from build123d import *

# Parameters (mm, degrees)
CROQUIS1_R              = 44
SALIENTE_EXTRUIR1_DEPTH = 20
CROQUIS3_R              = 2.1
CORTAR_EXTRUIR3_DEPTH   = 81.199750623
CORTAR_EXTRUIR5_DEPTH   = 3.5
VACIADO1_START          = 3
VACIADO1_DEPTH          = 17
VACIADO1_START_2        = 6.5
VACIADO1_2_DEPTH        = 13.5
CROQUIS2_R              = 3
CORTAR_EXTRUIR1_DEPTH   = 66.360538553
CROQUIS4_R              = 42.5
CORTAR_EXTRUIR4_DEPTH   = 2
CHAFL_N1_SIZE           = 2


# Read off the part's stored shape, not the designer's step: Vaciado1
with BuildPart() as part:
    # Croquis1 → Saliente-Extruir1 (new body)
    with BuildSketch(Plane(origin=(0, 0, 0), x_dir=(1, 0, 0), z_dir=(0, 1, 0))):
        with Locations(Location((0, 0, 0), (0, 0, 270))):
            Circle(CROQUIS1_R)
    extrude(amount=SALIENTE_EXTRUIR1_DEPTH)

    # Croquis3 → Cortar-Extruir3 (cut, through all)
    with BuildSketch(Plane(origin=(0, 20, -20), x_dir=(1, 0, 0), z_dir=(0, -1, 0))):
        with Locations(Location((-40, 20, 0), (0, 0, 270))):
            Circle(CROQUIS3_R)
        with Locations(Location((0, 60, 0), (0, 0, 270))):
            Circle(CROQUIS3_R)
        with Locations(Location((40, 20, 0), (0, 0, 270))):
            Circle(CROQUIS3_R)
        with Locations(Location((0, -20, 0), (0, 0, 270))):
            Circle(CROQUIS3_R)
    extrude(amount=CORTAR_EXTRUIR3_DEPTH, mode=Mode.SUBTRACT)

    # Croquis5 → Cortar-Extruir5 (cut)
    with BuildSketch(Plane.XZ):
        Polygon((40, -3.92598183), (43.4, -1.962990915), (43.4, 1.962990915), (40, 3.92598183), (36.6, 1.962990915), (36.6, -1.962990915), align=None)
        Polygon((3.92598183, 40), (1.962990915, 43.4), (-1.962990915, 43.4), (-3.92598183, 40), (-1.962990915, 36.6), (1.962990915, 36.6), align=None)
        Polygon((-3.92598183, -40), (-1.962990915, -43.4), (1.962990915, -43.4), (3.92598183, -40), (1.962990915, -36.6), (-1.962990915, -36.6), align=None)
        Polygon((-40, 3.92598183), (-43.4, 1.962990915), (-43.4, -1.962990915), (-40, -3.92598183), (-36.6, -1.962990915), (-36.6, 1.962990915), align=None)
    extrude(amount=-CORTAR_EXTRUIR5_DEPTH, mode=Mode.SUBTRACT)

    # Vaciado1 outline → Vaciado1 (cut)
    with BuildSketch(Plane(origin=(0, 0, 0), x_dir=(1, 0, 0), z_dir=(0, 1, 0)).offset(VACIADO1_START)):
        with BuildLine():
            ThreePointArc((-7.178364733, 40.366707567), (-28.991378029, 28.991378029), (-40.366707567, 7.178364733))
            Line((-40.366707567, 7.178364733), (-40, 7.390083446))
            Line((-40, 7.390083446), (-33.6, 3.695041723))
            Line((-33.6, 3.695041723), (-33.6, -3.695041723))
            Line((-33.6, -3.695041723), (-40, -7.390083446))
            Line((-40, -7.390083446), (-40.366707567, -7.178364733))
            ThreePointArc((-40.366707567, -7.178364733), (-28.991378029, -28.991378029), (-7.178364733, -40.366707567))
            Line((-7.178364733, -40.366707567), (-7.390083446, -40))
            Line((-7.390083446, -40), (-3.695041723, -33.6))
            Line((-3.695041723, -33.6), (3.695041723, -33.6))
            Line((3.695041723, -33.6), (7.390083446, -40))
            Line((7.390083446, -40), (7.178364733, -40.366707567))
            ThreePointArc((7.178364733, -40.366707567), (28.991378029, -28.991378029), (40.366707567, -7.178364733))
            Line((40.366707567, -7.178364733), (40, -7.390083446))
            Line((40, -7.390083446), (33.6, -3.695041723))
            Line((33.6, -3.695041723), (33.6, 3.695041723))
            Line((33.6, 3.695041723), (40, 7.390083446))
            Line((40, 7.390083446), (40.366707567, 7.178364733))
            ThreePointArc((40.366707567, 7.178364733), (28.991378029, 28.991378029), (7.178364733, 40.366707567))
            Line((7.178364733, 40.366707567), (7.390083446, 40))
            Line((7.390083446, 40), (3.695041723, 33.6))
            Line((3.695041723, 33.6), (-3.695041723, 33.6))
            Line((-3.695041723, 33.6), (-7.390083446, 40))
            Line((-7.390083446, 40), (-7.178364733, 40.366707567))
        make_face()
    extrude(amount=VACIADO1_DEPTH, mode=Mode.SUBTRACT)

    # Vaciado1 2 outline → Vaciado1 2 (cut)
    with BuildSketch(Plane(origin=(0, 0, 0), x_dir=(1, 0, 0), z_dir=(0, 1, 0)).offset(VACIADO1_START_2)):
        with BuildLine():
            ThreePointArc((-40.366707567, 7.178364733), (-40.540965383, 6.118016497), (-40.687375, 5.053465703))
            ThreePointArc((-40.687375, 5.053465703), (-34.9, 0), (-40.687375, -5.053465703))
            ThreePointArc((-40.687375, -5.053465703), (-40.540965383, -6.118016497), (-40.366707567, -7.178364733))
            Line((-40.366707567, -7.178364733), (-40, -7.390083446))
            Line((-40, -7.390083446), (-33.6, -3.695041723))
            Line((-33.6, -3.695041723), (-33.6, 3.695041723))
            Line((-33.6, 3.695041723), (-40, 7.390083446))
            Line((-40, 7.390083446), (-40.366707567, 7.178364733))
        make_face()
        with BuildLine():
            ThreePointArc((-5.053465703, 40.687375), (-6.118016497, 40.540965383), (-7.178364733, 40.366707567))
            Line((-7.178364733, 40.366707567), (-7.390083446, 40))
            Line((-7.390083446, 40), (-3.695041723, 33.6))
            Line((-3.695041723, 33.6), (3.695041723, 33.6))
            Line((3.695041723, 33.6), (7.390083446, 40))
            Line((7.390083446, 40), (7.178364733, 40.366707567))
            ThreePointArc((7.178364733, 40.366707567), (6.118016497, 40.540965383), (5.053465703, 40.687375))
            ThreePointArc((5.053465703, 40.687375), (0, 34.9), (-5.053465703, 40.687375))
        make_face()
        with BuildLine():
            Line((-7.390083446, -40), (-7.178364733, -40.366707567))
            ThreePointArc((-7.178364733, -40.366707567), (-6.118016497, -40.540965383), (-5.053465703, -40.687375))
            ThreePointArc((-5.053465703, -40.687375), (0, -34.9), (5.053465703, -40.687375))
            ThreePointArc((5.053465703, -40.687375), (6.118016497, -40.540965383), (7.178364733, -40.366707567))
            Line((7.178364733, -40.366707567), (7.390083446, -40))
            Line((7.390083446, -40), (3.695041723, -33.6))
            Line((3.695041723, -33.6), (-3.695041723, -33.6))
            Line((-3.695041723, -33.6), (-7.390083446, -40))
        make_face()
        with BuildLine():
            ThreePointArc((40.687375, 5.053465703), (40.540965383, 6.118016497), (40.366707567, 7.178364733))
            Line((40.366707567, 7.178364733), (40, 7.390083446))
            Line((40, 7.390083446), (33.6, 3.695041723))
            Line((33.6, 3.695041723), (33.6, -3.695041723))
            Line((33.6, -3.695041723), (40, -7.390083446))
            Line((40, -7.390083446), (40.366707567, -7.178364733))
            ThreePointArc((40.366707567, -7.178364733), (40.540965383, -6.118016497), (40.687375, -5.053465703))
            ThreePointArc((40.687375, -5.053465703), (34.9, 0), (40.687375, 5.053465703))
        make_face()
    extrude(amount=VACIADO1_2_DEPTH, mode=Mode.SUBTRACT)

    # Croquis2 → Cortar-Extruir1 (cut, through all)
    with BuildSketch(Plane.XZ):
        with Locations(Location((0, 25, 0), (0, 0, 270))):
            Circle(CROQUIS2_R)
        with Locations(Location((25, 0, 0), (0, 0, 270))):
            Circle(CROQUIS2_R)
        with Locations(Location((0, -25, 0), (0, 0, 270))):
            Circle(CROQUIS2_R)
        with Locations(Location((-25, 0, 0), (0, 0, 270))):
            Circle(CROQUIS2_R)
    extrude(amount=-CORTAR_EXTRUIR1_DEPTH, mode=Mode.SUBTRACT)

    # Croquis4 → Cortar-Extruir4 (cut)
    with BuildSketch(Plane(origin=(0, 20, 0), x_dir=(1, 0, 0), z_dir=(0, 1, 0))):
        with Locations(Location((0, 0, 0), (0, 0, 270))):
            Circle(CROQUIS4_R)
    extrude(amount=-CORTAR_EXTRUIR4_DEPTH, mode=Mode.SUBTRACT)

    # Chaflán1
    chafl_n1_edges = [part.edges().sort_by_distance(p)[0] for p in [
        (-28.991378029, 3, 28.991378029),
    ]]
    chamfer(chafl_n1_edges, length=CHAFL_N1_SIZE)


solid = part.part
Build history of the part. All positions in model axes, mm. A direction names the side the tool comes from. Round coordinates to 2 decimals unless told otherwise and drop trailing zeros. Loops run counter-clockwise (first coordinate to the right, second up) from the corner with the lowest first, then second, coordinate; pieces in that order, holes last. Notation, with made-up numbers: (37, -38.5) -> (54, -38.5) arc R22 ccw to (54, -20.5) -> close; hole circle Ø2 at (18.25, 53.25). An arc over 180 degrees is marked (long way). Answer in a Markdown table with one row per item.
Item 1: Saw through at C-C (z = -25). Write the cut outline in (x, y), and give its area (3 significant figures).
Answers below:
| item | result |
|---|---|
| outline | (-36.21, 0) -> (-3, 0) -> (-3, 3) -> (-32.5, 3) -> (-32.5, 18) -> (-34.37, 18) -> (-34.37, 20) -> (-36.21, 20) -> close; (3, 0) -> (36.21, 0) -> (36.21, 20) -> (34.37, 20) -> (34.37, 18) -> (32.5, 18) -> (32.5, 3) -> (3, 3) -> close |
| area | 318 mm² |
Item 2: Mould opens along Z. For faces 1 (the flat face through (23, 20, -36)), 2 (the flat face through (-5.568, 4.726, 36.845)) say: +Z half, -Z half, draft (parallel to the pull), parting line (faces both ways), or undercut.
Answers below:
| item | result |
|---|---|
| face 1 | draft |
| face 2 | undercut |
Item 3: Pin check, flat tips, straight feed: pin 1 (12 mm diameter, centred on x = 12.5, z = 3.5, fed in from +Y); pin 2 (4 mm diameter, centred on x = -34.5, y = 4, fed in from +Z); pin 3 (3 mm diameter, centred on y = 7, z = -26.5, fed in from -X). Stop position of each tip, or through.
Answers below:
| item | result |
|---|---|
| pin 1 | stops at y = 3 |
| pin 2 | stops at z = 29.66 |
| pin 3 | stops at x = -36.21 |
Item 4: Which spindle directions (+Z, -Z, +X, -X, +Y, -Y) get a long thin tool onto all of the face, cutting with end or side? Do faces 3 (the flat face through (36.845, 4.726, 5.568)), 4 (the cylindrical face through (25.9, 1.48, -2.86)), 5 (the flat face through (2.958, 1.726, -38.324)). Say none if no direction does.
Answers below:
| item | result |
|---|---|
| face 3 | +Y |
| face 4 | +Y, -Y |
| face 5 | -Y |
Item 5: Saw through at A-A (y = 12.25). Write the cut outline in (x, z).
Answers below:
| item | result |
|---|---|
| outline | circle Ø88 at (0, 0); hole circle Ø4.2 at (-40, 0); hole (-40.69, -5.05) arc R41 ccw to (-5.05, -40.69) arc R5.1 cw (long way) to (5.05, -40.69) arc R41 ccw to (40.69, -5.05) arc R5.1 cw (long way) to (40.69, 5.05) arc R41 ccw to (5.05, 40.69) arc R5.1 cw (long way) to (-5.05, 40.69) arc R41 ccw to (-40.69, 5.05) arc R5.1 cw (long way) to start; hole circle Ø4.2 at (0, -40); hole circle Ø4.2 at (0, 40); hole circle Ø4.2 at (40, 0) |
Item 6: Saw through at B-B (x = 25). Write the cut outline in (y, z).
Answers below:
| item | result |
|---|---|
| outline | (0, -36.21) -> (20, -36.21) -> (20, -34.37) -> (18, -34.37) -> (18, -32.5) -> (3, -32.5) -> (3, -3) -> (0, -3) -> close; (0, 3) -> (3, 3) -> (3, 32.5) -> (18, 32.5) -> (18, 34.37) -> (20, 34.37) -> (20, 36.21) -> (0, 36.21) -> close |
Item 7: Drill centre lines: L1, parallel to Z at x = -37, y = 6.25; L2, parallel to Z at x = -36.5, y = 6.25; L3, parallel to X at y = 18.75, z = 0. Where is each one in solid material? Low to high. Write a range as [from, to].
Answers below:
| item | result |
|---|---|
| L1 | z = [-23.81, -17.66], [-5.66, 5.66], [17.66, 23.81] |
| L2 | z = [-24.57, -18.67], [-5.37, 5.37], [18.67, 24.57] |
| L3 | x = [-44, -42.5], [42.5, 44] |
Item 8: Saw through at D-D (z = 0). State how many separate pieces and enclosed holes the cut face has, and give its area (3 significant figures).
Answers below:
| item | result |
|---|---|
| separate pieces | 5 |
| enclosed holes | 0 |
| area | 347 mm² |
